```python
from build123d import *

# Parameters (mm, degrees)
SKETCH1_W                             = 196.85
SKETCH1_H                             = 203.2
BOSS_EXTRUDE1_DEPTH                   = 0.7747
CUT_EXTRUDE7_DEPTH                    = 1.7747
SKETCH4_W                             = 196.85
SKETCH4_H                             = 0.6096
BOSS_EXTRUDE2_DEPTH                   = 12
SKETCH14_W                            = 196.85
SKETCH14_H                            = 11.938
BOSS_EXTRUDE3_DEPTH                   = 0.7747
SKETCH13_W                            = 196.85
SKETCH13_H                            = 0.6096
CUT_EXTRUDE9_DEPTH                    = 12
CSK_FOR_M3_FLAT_HEAD_MACHINE_SCREW3_D = 2.5
SKETCH19_W                            = 182.676330849
SKETCH19_H                            = 33.741187375
BOSS_EXTRUDE4_DEPTH                   = 0.7747
SKETCH21_W                            = 22.718000829
SKETCH21_H                            = 22.312299049
SKETCH21_W_2                          = 21.538835619
SKETCH21_H_2                          = 16.643270878
BOSS_EXTRUDE5_DEPTH                   = 0.7747
SKETCH22_W                            = 13.90531837
SKETCH22_H                            = 14.215216999
SKETCH22_W_2                          = 12.509578485
SKETCH22_H_2                          = 9.075576548
BOSS_EXTRUDE6_DEPTH                   = 0.7747


with BuildPart() as part:
    # Sketch1 → Boss-Extrude1 (new body)
    with BuildSketch(Plane(origin=(0, 0, 0), x_dir=(1, 0, 0), z_dir=(0, 0, -1))):
        with Locations((-104.775, 135.4)):
            Rectangle(SKETCH1_W, SKETCH1_H)
    extrude(amount=BOSS_EXTRUDE1_DEPTH)

    # Sketch2 → Cut-Extrude7 (cut, through all)
    with BuildSketch(Plane(origin=(0, 0, -0.7747), x_dir=(1, 0, 0), z_dir=(0, 0, -1))):
        with BuildLine():
            Line((-135.221253236, 173.5), (-135.221253236, 148))
            ThreePointArc((-135.221253236, 148), (-141.721253236, 141.5), (-148.221253236, 148))
            Line((-148.221253236, 148), (-148.221253236, 173.5))
            ThreePointArc((-148.221253236, 173.5), (-141.721253236, 180), (-135.221253236, 173.5))
        make_face()
        with BuildLine():
            Line((-62.069253236, 173.5), (-62.069253236, 148))
            ThreePointArc((-62.069253236, 148), (-68.569253236, 141.5), (-75.069253236, 148))
            Line((-75.069253236, 148), (-75.069253236, 173.5))
            ThreePointArc((-75.069253236, 173.5), (-68.569253236, 180), (-62.069253236, 173.5))
        make_face()
    extrude(amount=-CUT_EXTRUDE7_DEPTH, mode=Mode.SUBTRACT)

    # Sketch4 → Boss-Extrude2 (add)
    with BuildSketch(Plane.XY):
        with Locations((-104.775, -34.1048)):
            Rectangle(SKETCH4_W, SKETCH4_H)
    extrude(amount=BOSS_EXTRUDE2_DEPTH)

    # Sketch14 → Boss-Extrude3 (add)
    with BuildSketch(Plane.XY):
        with Locations((-104.775, -53.935004147)):
            Rectangle(SKETCH14_W, SKETCH14_H)
    extrude(amount=-BOSS_EXTRUDE3_DEPTH)

    # Sketch13 → Cut-Extrude9 (cut)
    with BuildSketch(Plane.XY.offset(12)):
        with Locations((-104.775, -34.1048)):
            Rectangle(SKETCH13_W, SKETCH13_H)
    extrude(amount=-CUT_EXTRUDE9_DEPTH, mode=Mode.SUBTRACT)

    # CSK for M3 Flat Head Machine Screw3 (through all)
    with Locations(Plane.XY):
        with Locations((-188.645, -72), (-188.645, -222), (-188.645, -197), (-188.645, -172), (-188.645, -147), (-188.645, -122), (-188.645, -97)):
            csk_for_m3_flat_head_machine_screw3 = Hole(CSK_FOR_M3_FLAT_HEAD_MACHINE_SCREW3_D / 2)

    # Mirror1: CSK for M3 Flat Head Machine Screw3 across plane
    add(csk_for_m3_flat_head_machine_screw3.mirror(Plane(origin=(-104.775, 0, 0), x_dir=(0, 0, 1), z_dir=(1, 0, 0))), mode=Mode.SUBTRACT)

    # Sketch19 → Boss-Extrude4 (add)
    with BuildSketch(Plane(origin=(0, 0, -0.7747), x_dir=(-1, 0, 0), z_dir=(0, 0, -1))):
        with Locations((101.266706015, -109.837466763)):
            Rectangle(SKETCH19_W, SKETCH19_H)
    extrude(amount=-BOSS_EXTRUDE4_DEPTH)

    # Sketch21 → Boss-Extrude5 (add)
    with BuildSketch(Plane(origin=(0, 0, -0.7747), x_dir=(-1, 0, 0), z_dir=(0, 0, -1))):
        with Locations((185.571692861, -170.919383368)):
            Rectangle(SKETCH21_W, SKETCH21_H)
        with Locations((24.271371833, -173.753897453)):
            Rectangle(SKETCH21_W_2, SKETCH21_H_2)
    extrude(amount=-BOSS_EXTRUDE5_DEPTH)

    # Sketch22 → Boss-Extrude6 (add)
    with BuildSketch(Plane.XY):
        with Locations((-189.313880795, -220.883843828)):
            Rectangle(SKETCH22_W, SKETCH22_H)
        with Locations((-23.670028487, -197.876391374)):
            Rectangle(SKETCH22_W_2, SKETCH22_H_2)
    extrude(amount=-BOSS_EXTRUDE6_DEPTH)


solid = part.part
```
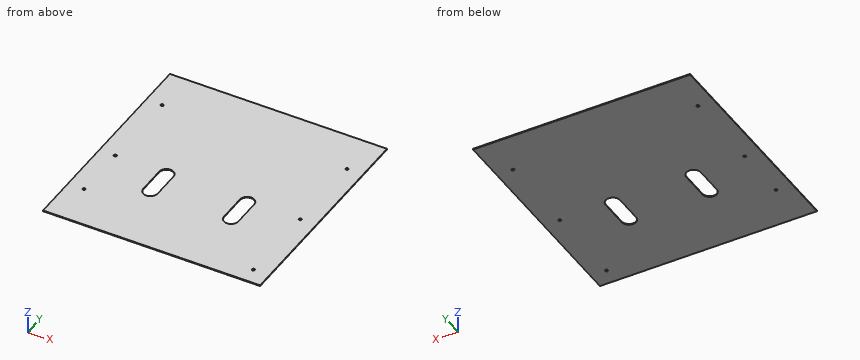
The model under review builds one solid part; all positions refer to its coordinate system, in mm. Round coordinates to 2 decimals unless told otherwise and drop trailing zeros. Write each loop counter-clockwise with the first axis right and the second up, starting at its lowest first coordinate (ties: lowest second). Pieces come first, ordered by that corner, then holes. Notation, with made-up numbers: (18, -31.5) - (70, -31.5) arc R10 ccw to (70, -17.5) - close; hole circle Ø6 at (28.25, -8). An arc over 180 degrees is marked (long way). Use one line per item in the form item = value.
Q1. Consider section B-B (y = -170). State the section outline as (x, z) points, and give its area (3 significant figures).
Answer key:
outline = (-203.2, -0.77) - (-148.22, -0.77) - (-148.22, 0) - (-203.2, 0) - close; (-135.22, -0.77) - (-75.07, -0.77) - (-75.07, 0) - (-135.22, 0) - close; (-62.07, -0.77) - (-6.35, -0.77) - (-6.35, 0) - (-62.07, 0) - close
area = 132 mm2
Q2. Consider section C-C (x = -142). State the section outline as (y, z) points, and give its area (3 significant figures).
Answer key:
outline = (-237, -0.77) - (-179.99, -0.77) - (-179.99, 0) - (-237, 0) - close; (-141.51, -0.77) - (-33.8, -0.77) - (-33.8, 0) - (-141.51, 0) - close
area = 128 mm2
Q3. Consider section A-A (z = -0.55). State how many separate pieces and enclosed holes the cut face has, and give its area (3 significant figures).
Answer key:
separate_pieces = 1
enclosed_holes = 8
area = 39,000 mm2
Q4. For line 1 (X direction, y = -72, z = -0.55) (3 decimals); line 2 (Y direction, x = -188.5, z = -0.35); line 3 (X direction, y = -155, z = -0.5), list the stretches that pass through material, from the lowest coordinate up. Write a range as [from, to].
Answer key:
line_1 = [-203.2, -189.895], [-187.395, -22.155], [-19.655, -6.35]
line_2 = [-237, -198.24], [-195.76, -148.24], [-145.76, -73.24], [-70.76, -33.8]
line_3 = [-203.2, -148.22], [-135.22, -75.07], [-62.07, -6.35]
